Design review of the part built by this model. Coordinates are the model's own, in mm. Face numbers are marked on the shaded views. Coordinates: 2 decimals unless noted, no trailing zeros. Write each loop counter-clockwise with the first axis right and the second up, starting at its lowest first coordinate (ties: lowest second). Pieces come first, ordered by that corner, then holes. Notation, with made-up numbers: M 76.5,55 L 111.5,55 A11 ccw 111.5,63 Z; hole C 83.5,41 d4. An arc over 180 degrees is marked long. Return JSON: item names as keys, results as strings. Group by question number.
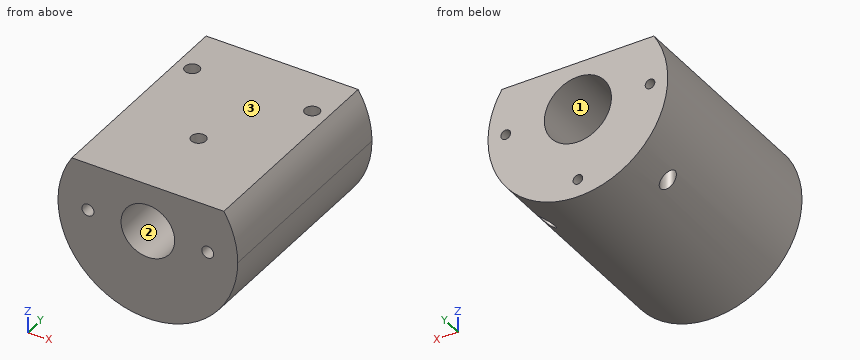
```python
from build123d import *

# Parameters (mm, degrees)
SKETCH1_R             = 2
SKETCH1_R_2           = 14
SKETCH1_R_3           = 11.2
BOSS_EXTRUDE1_DEPTH   = 90
SKETCH1_3_R           = 2
CORTE_EXTRUS_O1_DEPTH = 14.6
SKETCH1_4_R           = 14
SKETCH1_4_R_2         = 11.2
CORTE_EXTRUS_O2_DEPTH = 50
ESBO_O1_R             = 2.5
CORTE_EXTRUS_O3_DEPTH = 23
ESBO_O2_R             = 3.05
CORTE_EXTRUS_O4_DEPTH = 58.5
CORTE_EXTRUS_O5_REACH = 59.5
ESBO_O2_3_R           = 3.05


with BuildPart() as part:
    # Sketch1 → Boss-Extrude1 (new body)
    with BuildSketch(Plane(origin=(0, 0, 0), x_dir=(1, 0, 0), z_dir=(0, 1, 0))):
        with BuildLine():
            ThreePointArc((37.5, 0), (-10.409031069, 36.026407984), (-31.721443851, -20))
            Line((-31.721443851, -20), (31.721443851, -20))
            ThreePointArc((31.721443851, -20), (36.026407984, -10.409031069), (37.5, 0))
        make_face()
        with Locations((-30.1, 0)):
            Circle(SKETCH1_R, mode=Mode.SUBTRACT)
        Circle(SKETCH1_R_2, mode=Mode.SUBTRACT)
        with Locations((30.1, 0)):
            Circle(SKETCH1_R, mode=Mode.SUBTRACT)
        with Locations((0, 30.1)):
            Circle(SKETCH1_R, mode=Mode.SUBTRACT)
        Circle(SKETCH1_R_2)
        Circle(SKETCH1_R_3, mode=Mode.SUBTRACT)
        with Locations((-30.1, 0)):
            Circle(SKETCH1_R)
        with Locations((0, 30.1)):
            Circle(SKETCH1_R)
        with Locations((30.1, 0)):
            Circle(SKETCH1_R)
    extrude(amount=-BOSS_EXTRUDE1_DEPTH)

    # Sketch1_3 → Corte-extrus_o1 (cut)
    with BuildSketch(Plane(origin=(0, 0, 0), x_dir=(1, 0, 0), z_dir=(0, 1, 0))):
        with Locations((-30.1, 0)):
            Circle(SKETCH1_3_R)
        with Locations((0, 30.1)):
            Circle(SKETCH1_3_R)
        with Locations((30.1, 0)):
            Circle(SKETCH1_3_R)
    extrude(amount=-CORTE_EXTRUS_O1_DEPTH, mode=Mode.SUBTRACT)

    # Sketch1_4 → Corte-extrus_o2 (cut)
    with BuildSketch(Plane(origin=(0, 0, 0), x_dir=(1, 0, 0), z_dir=(0, 1, 0))):
        Circle(SKETCH1_4_R)
        Circle(SKETCH1_4_R_2, mode=Mode.SUBTRACT)
    extrude(amount=-CORTE_EXTRUS_O2_DEPTH, mode=Mode.SUBTRACT)

    # Esbo_o1 → Corte-extrus_o3 (cut)
    with BuildSketch(Plane.XZ.offset(90)):
        with Locations((-25, 0)):
            Circle(ESBO_O1_R)
        with Locations((25, 0)):
            Circle(ESBO_O1_R)
    extrude(amount=-CORTE_EXTRUS_O3_DEPTH, mode=Mode.SUBTRACT)

    # Esbo_o2 → Corte-extrus_o4 (cut, through all)
    with BuildSketch(Plane.XY.offset(20)):
        with Locations((25.05, -20.05)):
            Circle(ESBO_O2_R)
        with Locations((-25.05, -20.05)):
            Circle(ESBO_O2_R)
    extrude(amount=-CORTE_EXTRUS_O4_DEPTH, mode=Mode.SUBTRACT)

    # Esbo_o2_3 → Corte-extrus_o5 (cut, up to next)
    with BuildSketch(Plane.XY.offset(20), mode=Mode.PRIVATE) as corte_extrus_o5_sk1:
        with Locations((0, -55.95)):
            Circle(ESBO_O2_3_R)
    corte_extrus_o5_tool1 = extrude(corte_extrus_o5_sk1.sketch, amount=-CORTE_EXTRUS_O5_REACH, mode=Mode.PRIVATE) & part.part
    add(corte_extrus_o5_tool1.solids().sort_by_distance((0, -55.95, 20))[0], mode=Mode.SUBTRACT)


solid = part.part
```
Item 1: The part is to be moulded in two halves that separate along X. For the marked faces 1, 2 and 3, say which applies: pulls with the +X half, pulls with the -X half, needs draft (parallel to the pull), parting line crosses it, or undercut.
Item 2: For line 1 (X direction, y = -10.5, z = 0); line 2 (Z direction, x = 0, y = -10); line 3 (Y direction, x = -25, z = 15.5), list the stretches that pass through material, from the lowest coordinate up.
Item 3: Add section A-A (y = -20.05). Write out the cut boundary in (x, z), plus the area to 3 significant figures.
Item 4: For pin 1 (14 mm diameter, centred on x = -2, z = 2, fed in from +Y); pin 2 (2.5 mm diameter, centred on x = 25.5, z = -1, fed in from -Y); pin 3 (2.5 mm diameter, centred on x = 30.1, z = 0, fed in from +Y); pin 4 (3 mm diameter, centred on x = -13, y = -72, fed in from -Z), all flat-tipped, find the tip position at first contact; note any pin that passes through.
Item 5: Add section D-D (y = -10). Write out the cut boundary in (x, z).
Item 6: Add section C-C (y = -80.5). Write out the cut boundary in (x, z), plus the area to 3 significant figures.
Item 7: Add section B-B (x = 6.5). Write out the cut boundary in (y, z).
Geometry check:
{
 "1": {"face 1": "undercut", "face 2": "undercut", "face 3": "needs draft"},
 "2": {"line 1": "-37.5 to -32.1, -28.1 to -14, 14 to 28.1, 32.1 to 37.5", "line 2": "-37.5 to -32.1, -28.1 to -14, 14 to 20", "line 3": "-90 to -23.1, -17 to 0"},
 "3": {"outline": "M -31.72,20 A37.5 ccw -28.1,-24.83 L -28.1,20 Z; M -22,-30.37 A37.5 ccw 22,-30.37 L 22,20 L -22,20 Z; M 28.1,-24.83 A37.5 ccw 31.72,20 L 28.1,20 Z; hole C 0,0 d28", "area": "2,440 mm^2"},
 "4": {"pin 1": "through", "pin 2": "y = -67", "pin 3": "y = -14.6", "pin 4": "z = -35.69"},
 "5": {"outline": "M -31.72,20 A37.5 ccw long 31.72,20 Z; hole C -30.1,0 d4; hole C 0,0 d28; hole C 0,-30.1 d4; hole C 30.1,0 d4"},
 "6": {"outline": "M -31.72,20 A37.5 ccw long 31.72,20 Z; hole C -25,0 d5; hole C 0,0 d22.4; hole C 25,0 d5", "area": "3,200 mm^2"},
 "7": {"outline": "M -90,-36.93 L 0,-36.93 L 0,-12.4 L -50,-12.4 L -50,-9.12 L -90,-9.12 Z; M -90,9.12 L -50,9.12 L -50,12.4 L 0,12.4 L 0,20 L -90,20 Z"}
}
